The listing builds one solid part. Answer for the finished solid, in the listing's coordinates (mm). A direction names the side the tool comes from. Coordinates: 2 decimals unless noted, no trailing zeros. Order: outer loops, then holes, each group sorted by start corner. A loop starts at its lowest first (then second) coordinate and runs counter-clockwise, first axis right, second up. Notation, with made-up numbers: (52, 89) - (82, 89) arc R8 cw to (82, 93) - close; hole circle Ø4 at (-36, 20). An arc over 180 degrees is marked (long way). Use one line per item in the form item = value. Start each with the question number.
Item 1: A tool of negligible diameter and unlimited length cuts with its end or side. For faces 1 (the flat face through (-29, 12.5, 10)), 2 (the flat face through (-31, 0, 22)), from which of +Z, -Z, +X, -X, +Y, -Y can it reach the whole face along a straight path? Write none if from no direction.
Item 2: Each of these flat-tipped pins is pushed along its axis until it touches: pin 1 Ø1 at (x, z) = (-9.5, 8.5) entering from -Y; pin 2 Ø2 at (x, z) = (-19.5, 19.5) entering from -Y; pin 3 Ø3.5 at (y, z) = (-8, 11) entering from -X; pin 4 Ø2.5 at (x, y) = (-35, 0) entering from -Z. Where does it stop, or does it pass through?
Item 3: The mould has two halves that part along Z. Classify faces 3 (the cylindrical face through (-43.732, -9.474, 12.352)), 4 (the flat face through (-9.873, -6.337, 9.614)), 5 (the cylindrical face through (-8.403, -6.387, 20.496)): released by +Z, released by -Z, zero draft, split by the parting line, or undercut.
Item 4: Section B-B, the plane z = 3.25 is taken. Write down the section's boundary in (x, y).
Item 5: Section D-D, the plane x = -26 is taken. Write down the section's boundary in (y, z), and give its area (3 significant figures).
Item 6: Section A-A, the plane x = -35 is taken. Write down the section's boundary in (y, z).
Item 7: Section C-C, the plane z = 11 is taken. Count the separate pieces of the cut face and the enclosed holes in it, and give its area (3 significant figures).
Item 8: Consider line 1 along Y through (x, z) = (-35, 12.75); line 2 along Z through (x, y) = (-43.9, 8); line 3 along Y through (x, z) = (-22, 3.5). Determine where each line is inside the solid, lowest interval first. Write a range as [from, to].
from build123d import *

# Parameters (mm, degrees)
F1_DEPTH = 22
F2_D     = 4
F3_T     = -2.5
F5_D     = 4
F5_DEPTH = 6
F5_TIP   = 1.2017212381
F6_R     = 4.99999


# Not quite as in the source:
# - a fillet or chamfer is up to 0.001 mm smaller than in the source, because OpenCascade refuses the exact size


with BuildPart() as f1:
    # F0 (on Top) → F1 (new body)
    with BuildSketch(Plane.XY):
        Polygon((-15, -15), (0, 0), (-15, 15), (-45, 15), (-45, -15), align=None)
    extrude(amount=F1_DEPTH)

    # F2 (through all)
    with Locations(Plane(origin=(0, 0, 0), x_dir=(1, 0, 0), z_dir=(0, 0, -1))):
        with Locations((-35, 0), (-10, 0)):
            Hole(F2_D / 2)

    # F3
    f3_openings = [f1.faces().sort_by_distance(p)[0] for p in [
        (-26.079977, 0, 0),
    ]]
    offset(amount=F3_T, openings=f3_openings)

    # F5
    with Locations(Plane(origin=(-45, 0, 0), x_dir=(0, -1, 0), z_dir=(-1, 0, 0))):
        with Locations((-8, 11), (8, 11)):
            Hole(F5_D / 2, depth=F5_DEPTH)
            with Locations((0, 0, -(F5_DEPTH + F5_TIP / 2))):  # 118° drill point
                Cone(0, F5_D / 2, F5_TIP, mode=Mode.SUBTRACT)

    # F6 (radius 5 in the source; OpenCascade refuses exactly that, so slightly less here)
    f6_edges = [f1.edges().sort_by_distance(p)[0] for p in [
        (-30, -15, 22),
        (-7.5, -7.5, 22),
        (-7.5, 7.5, 22),
        (-30, 15, 22),
        (-45, 15, 11),
        (-45, -15, 11),
    ]]
    fillet(f6_edges, radius=F6_R)


solid = f1.part
Response:
q1.face_1 = -Z
q1.face_2 = +Z, +X, -X, +Y, -Y
q2.pin_1 = -10
q2.pin_2 = -14.77
q2.pin_3 = -13.29
q2.pin_4 = through
q3.face_3 = undercut
q3.face_4 = zero draft
q3.face_5 = released by +Z
q4.outline = (-45, -10) arc R5 ccw to (-40, -15) - (-15, -15) - (0, 0) - (-15, 15) - (-40, 15) arc R5 ccw to (-45, 10) - close; circle Ø9 at (-35, 0); circle Ø9 at (-10, 0); hole (-42.5, -12.5) - (-16.04, -12.5) - (-3.54, 0) - (-16.04, 12.5) - (-42.5, 12.5) - close; hole circle Ø4 at (-35, 0); hole circle Ø4 at (-10, 0)
q5.outline = (-15, 0) - (-12.5, 0) - (-12.5, 19.5) - (12.5, 19.5) - (12.5, 0) - (15, 0) - (15, 17) arc R5 ccw to (10, 22) - (-10, 22) arc R5 ccw to (-15, 17) - close
q5.area = 162 mm2
q6.outline = (-15, 0) - (-12.5, 0) - (-12.5, 19.5) - (-4.5, 19.5) - (-4.5, 0) - (-2, 0) - (-2, 22) - (-10, 22) arc R5 ccw to (-15, 17) - close; (2, 0) - (4.5, 0) - (4.5, 19.5) - (12.5, 19.5) - (12.5, 0) - (15, 0) - (15, 17) arc R5 ccw to (10, 22) - (2, 22) - close
q7.separate_pieces = 4
q7.enclosed_holes = 2
q7.area = 379 mm2
q8.line_1 = [-15, -12.5], [-4.5, -2], [2, 4.5], [12.5, 15]
q8.line_2 = [0, 9], [13, 22]
q8.line_3 = [-15, -12.5], [12.5, 15]
